from build123d import *

# Parameters (mm, degrees)
SKETCH1_R           = 14
SKETCH1_R_2         = 6
SKETCH1_R_3         = 1.6
BOSS_EXTRUDE1_DEPTH = 4
CUT_EXTRUDE1_REACH  = 6


with BuildPart() as part:
    # Sketch1 → Boss-Extrude1 (new body)
    with BuildSketch(Plane.XZ.offset(-7.168741666)):
        with Locations((7.114749013, 17.625339305)):
            Circle(SKETCH1_R)
        with Locations((7.114749013, 17.625339305)):
            Circle(SKETCH1_R_2, mode=Mode.SUBTRACT)
        with Locations((2.364749013, 25.852580641)):
            Circle(SKETCH1_R_3, mode=Mode.SUBTRACT)
        with Locations((-2.385250987, 17.625339305)):
            Circle(SKETCH1_R_3, mode=Mode.SUBTRACT)
        with Locations((2.364749013, 9.398097969)):
            Circle(SKETCH1_R_3, mode=Mode.SUBTRACT)
        with Locations((11.864749013, 9.398097969)):
            Circle(SKETCH1_R_3, mode=Mode.SUBTRACT)
        with Locations((16.614749013, 17.625339305)):
            Circle(SKETCH1_R_3, mode=Mode.SUBTRACT)
        with Locations((11.864749013, 25.852580641)):
            Circle(SKETCH1_R_3, mode=Mode.SUBTRACT)
    extrude(amount=BOSS_EXTRUDE1_DEPTH)

    # Sketch2 → Cut-Extrude1 (cut, up to next)
    with BuildSketch(Plane.XZ.offset(-3.168741666), mode=Mode.PRIVATE) as cut_extrude1_sk1:
        Polygon((11.864749013, 7.798097969), (2.364749013, 7.798097969), (1.133638883, 10.420041142), (3.282462114, 13.008676319), (10.947035911, 13.008676319), (13.095859142, 10.420041142), align=None)
    cut_extrude1_tool1 = extrude(cut_extrude1_sk1.sketch, amount=-CUT_EXTRUDE1_REACH, mode=Mode.PRIVATE) & part.part
    add(cut_extrude1_tool1.solids().sort_by_distance((7.114749, 3.168742, 10.326739))[0], mode=Mode.SUBTRACT)
    # Sketch2 → Cut-Extrude1 (cut, up to next)
    with BuildSketch(Plane.XZ.offset(-3.168741666), mode=Mode.PRIVATE) as cut_extrude1_sk2:
        Polygon((1.133638883, 24.830637468), (2.364749013, 27.452580641), (11.864749013, 27.452580641), (13.095859142, 24.830637468), (10.947035911, 22.242002291), (3.282462114, 22.242002291), align=None)
    cut_extrude1_tool2 = extrude(cut_extrude1_sk2.sketch, amount=-CUT_EXTRUDE1_REACH, mode=Mode.PRIVATE) & part.part
    add(cut_extrude1_tool2.solids().sort_by_distance((7.114749, 3.168742, 24.923939))[0], mode=Mode.SUBTRACT)


solid = part.part
Could you check a few things on this model? Use its own coordinates, in mm. A direction names the side the tool comes from. Give positions to 0.01 mm unless a question says otherwise; leave off trailing zeros. Order: outer loops, then holes, each group sorted by start corner. A loop starts at its lowest first (then second) coordinate and runs counter-clockwise, first axis right, second up.
Item 1: If we section it at D-D, the plane z = 29: Write out the boundary of the cut face in (x, y), plus the area to 3 significant figures.
Item 2: If we section it at C-C, the plane y = 5.8: Write out the boundary of the cut face in (x, z), plus the area to 3 significant figures.
Item 3: I'm going to push flat-ended pins straight in: pin 1 (1 mm diameter, centred on x = 2, y = 4, fed in from +Z); pin 2 (1 mm diameter, centred on x = 9.5, y = 5.5, fed in from +Z); pin 3 (1.2 mm diameter, centred on x = 9.5, y = 4.5, fed in from -Z). Where does each tip first touch, or does it pass through?
Item 4: I need wall thicknesses on line 1 (Z direction, x = 3, y = 4.1); line 2 (Z direction, x = 7.5, y = 4.3); line 3 (Z direction, x = 1.75, y = 4.05). Which ranges of each line are inside material? Lowest first, please.
Item 5: If we mould it in two halves opening along Z, with no side actions, what happens to faces 1 (the face through (5.292, 5.197, 31.506)), 2 (the face through (13, 3.169, 15)), 3 (the face through (13.302, 5.197, 8.695))? For each: pulls with the +Z half, pulls with the -Z half, needs draft (parallel to the pull), parting line crosses it, or undercut.
Item 6: For faces 4 (the face through (13.114, 5.197, 17.552)), 5 (the face through (13, 7.169, 15)), which set-ups out of +Z, -Z, +X, -X, +Y, -Y let a thin tool reach every point of the face, with its end or its side?
Item 7: If we section it at B-B, the plane z = 14.5: Write out the boundary of the cut face in (x, y).
Item 8: If we section it at A-A, the plane x = 5: Write out the boundary of the cut face in (y, z).
Values:
1. outline: (-1.05, 3.17) - (15.28, 3.17) - (15.28, 7.17) - (-1.05, 7.17) - close
1. area: 65.3 mm2
2. outline: circle Ø28 at (7.11, 17.63); hole circle Ø3.2 at (-2.39, 17.63); hole (1.13, 10.42) arc R1.6 ccw to (2.36, 7.8) - (11.86, 7.8) arc R1.6 ccw to (13.1, 10.42) - (10.95, 13.01) arc R6 ccw to (10.95, 22.24) - (13.1, 24.83) arc R1.6 ccw to (11.86, 27.45) - (2.36, 27.45) arc R1.6 ccw to (1.13, 24.83) - (3.28, 22.24) arc R6 ccw to (3.28, 13.01) - close; hole circle Ø3.2 at (16.61, 17.63)
2. area: 386 mm2
3. pin 1: stops at z = 30.84
3. pin 2: stops at z = 31.5
3. pin 3: stops at z = 3.74
4. line 1: z = 4.24 to 7.8, 12.67 to 13.26, 21.99 to 22.58, 27.45 to 31.01
4. line 2: z = 3.63 to 7.8, 27.45 to 31.62
4. line 3: z = 4.69 to 7.92, 11.16 to 14.94, 20.31 to 24.09, 27.33 to 30.56
5. face 1: parting line crosses it
5. face 2: needs draft
5. face 3: undercut
6. face 4: +Y, -Y
6. face 5: +Z, -Z, +X, -X, +Y
7. outline: (-6.53, 3.17) - (1.99, 3.17) - (1.99, 7.17) - (-6.53, 7.17) - close; (12.24, 3.17) - (20.76, 3.17) - (20.76, 7.17) - (12.24, 7.17) - close
8. outline: (3.17, 3.79) - (7.17, 3.79) - (7.17, 7.8) - (3.17, 7.8) - close; (3.17, 27.45) - (7.17, 27.45) - (7.17, 31.46) - (3.17, 31.46) - close
